Geometry check sheet. Reference: the model listing, model coordinates, mm. Face numbers are marked on the shaded views. Give positions to 0.01 mm unless a question says otherwise; leave off trailing zeros. Write item = value, one per line. Start each with the question number.
from build123d import *

# Parameters (mm, degrees)
SKETCH11_W          = 81
SKETCH11_H          = 81
BOSS_EXTRUDE1_DEPTH = 27


with BuildPart() as part:
    # Sketch11 → Boss-Extrude1 (new body)
    with BuildSketch(Plane(origin=(0, 0, 0), x_dir=(1, 0, 0), z_dir=(0, 1, 0))):
        Rectangle(SKETCH11_W, SKETCH11_H)
    extrude(amount=BOSS_EXTRUDE1_DEPTH)

    # Sketch1 → Cut-Revolve1 (revolve, cut)
    with BuildSketch(Plane.XY):
        with BuildLine():
            Line((0, 25), (0, 10))
            Line((0, 10), (0, -10))
            Line((0, -10), (31.5, -10))
            Line((31.5, -10), (31.5, 0))
            add(Edge.make_bspline(
                [(0, 25), (1.37149288, 25), (4.090224786, 24.302680674), (10.751491586, 17.136812446), (25.578767024, 15.070162158), (31.038481607, 6.450242929), (31.5, 0)],
                knots=[0, 0, 0, 0, 0.091245862, 0.195023315, 0.675457006, 1, 1, 1, 1], degree=3))
        make_face()
    revolve(axis=Axis((0, 10, 0), (0, -1, 0)), mode=Mode.SUBTRACT)


solid = part.part
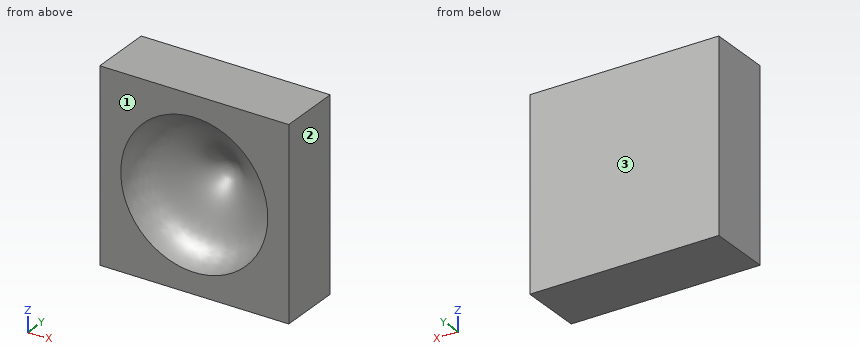
1) Gauge pin test, flat ends, axial feed: P1, Ø1.5, axis at x = 18.5, z = -7, coming from the -Y side; P2, Ø1, axis at x = 16, z = 11.5, coming from the -Y side. Record the tip position at first contact, or that the pin passes through.
2) Release check for a two-part mould opening along Y. For the marked faces 1, 2 and 3 record: pulls with the +Y half, pulls with the -Y half, needs draft (parallel to the pull), parting line crosses it, or undercut.
3) Material ranges on line 1 along Z through (x, y) = (-16.5, 2); line 2 along Z through (x, y) = (-1, 12.5); line 3 along X through (y, z) = (7.25, -9.5), recorded low to high.
Checked values:
q1.P1 = 14.82
q1.P2 = 14.96
q2.face_1 = pulls with the -Y half
q2.face_2 = needs draft
q2.face_3 = pulls with the +Y half
q3.line_1 = -40.5 to -26.58, 26.58 to 40.5
q3.line_2 = -40.5 to -25.07, 25.07 to 40.5
q3.line_3 = -40.5 to -28.22, 28.22 to 40.5
